Design review of the part built by this model. Coordinates are the model's own, in mm. A direction names the side the tool comes from. Round coordinates to 2 decimals unless told otherwise and drop trailing zeros. Loops run counter-clockwise (first coordinate to the right, second up) from the corner with the lowest first, then second, coordinate; pieces in that order, holes last. Notation, with made-up numbers: (9, -8.75) - (22, -8.75) arc R27 ccw to (22, 21.25) - close; hole circle Ø8 at (-31.75, 7). An arc over 180 degrees is marked (long way). Return JSON: item names as keys, results as strings. Group by question number.
(1) Clearance check with flat-ended pins moving along their axes: pin 1 (6.5 mm diameter, centred on x = 0, z = 25, fed in from -Y); pin 2 (2 mm diameter, centred on x = -1.5, z = 24.5, fed in from +Y); pin 3 (12 mm diameter, centred on x = 2.5, z = 10.5, fed in from -Y); pin 4 (3.5 mm diameter, centred on y = 120, z = 30, fed in from -X). State where each tip first meets the part, or that it passes through.
(2) Wall thickness on L1, parallel to Z at x = 0, y = 295; L2, parallel to Z at x = -5, y = 220; L3, parallel to Y at x = 1.5, z = -30: over which ranges is each line inside the solid? List them lowest first. Write a range as [from, to].
(3) For faces 1 (the flat face through (-10, 148, -1)), 2 (the flat face through (0, 288, -25)), 3 (the flat face through (0, 12, -25)), list the 3-axis set-ups (+Z, -Z, +X, -X, +Y, -Y) from which the entire face can be reached by the end or side of a thin tool; tool diameter is ignored.
(4) We need section A-A, the plane z = 25. Write out the cut boundary in (x, y).
(5) The part is to be moulded in two halves that separate along X. For faces 4 (the flat face through (0, 148, 40)), 5 (the flat face through (10, 148, 1)), 6 (the cylindrical face through (-0.46, 5.92, 28.47)), say which applies: pulls with the +X half, pulls with the -X half, needs draft (parallel to the pull), parting line crosses it, or undercut.
Autodesk Inventor part; units mm, degrees
ref_plane "YZ Plane" through (0, 0, 0) normal (1, 0, 0) x (0, 1, 0)
ref_plane "XZ Plane" through (0, 0, 0) normal (0, 1, 0) x (-1, 0, 0)
ref_plane "XY Plane" through (0, 0, 0) normal (0, 0, 1) x (1, 0, 0)
sketch "Sketch1" plane through (0, 0, 0) normal (0, 1, 0) x (-1, 0, 0)
  line L0 (10, 40) -> (-10, 40)
  line L1 (-10, 40) -> (-10, -40)
  line L2 (-10, -40) -> (10, -40)
  line L3 (10, -40) -> (10, 40)
  line L4 (10, 0) -> (-10, 0) construction
  line L5 (0, 40) -> (0, -40) construction
  point P0 (0, 0)
  point P1 (0, 0)
  dimension "d0" = 20
  dimension "d1" = 80
extrude "Extrusion1" add sketch "Sketch1" along normal blind 300
sketch "Sketch2" plane through (0, 300, 0) normal (0, 1, 0) x (1, 0, 0)
  circle A0 centre (0, 25) radius 3.5
  circle A1 centre (0, -25) radius 3.5
  line L0 (0, -25) -> (0, 25) construction
  line L1 (10, 40) -> (-10, 40) construction
  line L2 (0, 40) -> (0, -40) construction
  line L3 (-10, -40) -> (10, -40) construction
  point P0 (0, 0)
  dimension "d4" = 7
  dimension "d5" = 7
  dimension "d6" = 50
  dimension "d7" = 15
extrude "Extrusion2" cut sketch "Sketch2" against normal blind 12
sketch "Sketch3" plane through (0, 0, 0) normal (0, -1, 0) x (1, 0, 0)
  circle A0 centre (0, 25) radius 3.5
  circle A1 centre (0, -25) radius 3.5
  point P0 (0, 0)
extrude "Extrusion3" cut sketch "Sketch3" against normal blind 12
sketch "Sketch4" plane through (-10, 0, -40) normal (-1, 0, 0) x (0, 0, 1)
  circle A0 centre (10, 120) radius 2.25
  circle A1 centre (70, 120) radius 2.25
  line L0 (10, 120) -> (70, 120) construction
  line L1 (0, 0) -> (0, 300) construction
  line L2 (0, 0) -> (80, 0) construction
  point P0 (40, 0)
  dimension "d12" = 4.5
  dimension "d13" = 4.5
  dimension "d14" = 60
  dimension "d15" = 10
  dimension "d16" = 120
extrude "Extrusion4" cut sketch "Sketch4" against normal up to next
sketch "Sketch5" plane through (-10, 0, -40) normal (-1, 0, 0) x (0, 0, 1)
  circle A0 centre (30, 220) radius 1.75
  circle A1 centre (50, 220) radius 1.75
  line L0 (30, 220) -> (50, 220) construction
  line L1 (0, 0) -> (0, 300) construction
  line L2 (0, 300) -> (80, 300) construction
  point P0 (40, 0)
  dimension "d19" = 3.5
  dimension "d20" = 3.5
  dimension "d21" = 20
  dimension "d22" = 30
  dimension "d23" = 80
extrude "Extrusion5" cut sketch "Sketch5" against normal up to next
properties part number "side_panel"
Solutions:
{
 "1": {"pin 1": "y = 12", "pin 2": "y = 288", "pin 3": "y = 0", "pin 4": "through"},
 "2": {"L1": "[-40, -28.5], [-21.5, 21.5], [28.5, 40]", "L2": "[-40, -11.75], [-8.25, 8.25], [11.75, 40]", "L3": "[0, 117.75], [122.25, 300]"},
 "3": {"face 1": "+Z, -Z, -X, +Y, -Y", "face 2": "+Y", "face 3": "-Y"},
 "4": {"outline": "(-10, 0) - (-3.5, 0) - (-3.5, 12) - (3.5, 12) - (3.5, 0) - (10, 0) - (10, 300) - (3.5, 300) - (3.5, 288) - (-3.5, 288) - (-3.5, 300) - (-10, 300) - close"},
 "5": {"face 4": "needs draft", "face 5": "pulls with the +X half", "face 6": "undercut"}
}
